Autodesk Inventor part; units mm, degrees
ref_plane "YZ Plane" through (0, 0, 0) normal (1, 0, 0) x (0, 1, 0)
ref_plane "XZ Plane" through (0, 0, 0) normal (0, 1, 0) x (-1, 0, 0)
ref_plane "XY Plane" through (0, 0, 0) normal (0, 0, 1) x (1, 0, 0)
sketch "スケッチ1" plane through (0, 0, 0) normal (0, 0, 1) x (1, 0, 0)
  circle A0 centre (0, 0) radius 3
  circle A1 centre (0, 40) radius 1.25
  circle A2 centre (0, 40) radius 3
  circle A3 centre (0, 0) radius 5
  line L0 (0, 5) -> (0, 37)
  line L1 (-2.9962, 40.15) -> (-4.9937, 0.25)
  dimension "d0" = 6
  dimension "d1" = 2.5
  dimension "d2" = 40
  dimension "d3" = 6
  dimension "d4" = 10
extrude "押し出し1" add sketch "スケッチ1" along normal blind 3
sketch "スケッチ2" plane through (0, 0, 3) normal (0, 0, 1) x (1, 0, 0)
  circle A0 centre (0, 0) radius 3
  circle A1 centre (0, 40) radius 1.25
  arc A2 (0, 37) -> (-2.9962, 40.15) centre (0, 40) ccw
  line L0 (-2.9962, 40.15) -> (-4.9937, 0.25)
  arc A3 (-4.9937, 0.25) -> (0, 5) centre (0, 0) ccw
  line L1 (0, 5) -> (0, 37)
  circle A4 centre (0, 0) radius 3
  circle A5 centre (-32.1289, 23.8272) radius 1.25
  line L2 (-4.0161, 2.9784) -> (-4.827, 3.5798)
  arc A6 (-30.4645, 26.3232) -> (-29.7192, 22.0402) centre (-32.1289, 23.8272) ccw
  line L3 (-4.5534, 9.0458) -> (2.7739, 4.16)
  arc A7 (-4.0161, 2.9784) -> (2.7739, 4.16) centre (0, 0) ccw
extrude "押し出し2" [suppressed]
sketch "スケッチ4" plane through (0, 0, 3) normal (0, 0, 1) x (1, 0, 0)
  line L0 (-4.9937, 0.25) -> (-2.9962, 40.15)
  arc A0 (0, 37) -> (-2.9962, 40.15) centre (0, 40) ccw
  line L1 (0, 37) -> (0, 5)
  circle A1 centre (0, 40) radius 1.25
  circle A2 centre (-27.9404, 11.376) radius 3
  circle A3 centre (0, 40) radius 1.25
  line L2 (-3.1661, 36.7564) -> (-2.0955, 37.8532)
  arc A4 (2.2489, 38.0144) -> (-2.0955, 37.8532) centre (0, 40) ccw
  line L3 (2.2489, 38.0144) -> (-3.4249, 31.5882)
  arc A5 (-24.4479, 14.954) -> (-24.1923, 8.0667) centre (-27.9404, 11.376) ccw
  circle A6 centre (0, 0) radius 3
  arc A7 (-4.9937, 0.25) -> (0, 5) centre (0, 0) ccw
extrude "押し出し3" [suppressed]
sketch "スケッチ5" plane through (0, 0, 3) normal (0, 0, 1) x (1, 0, 0)
  circle A0 centre (0, 0) radius 3
  circle A1 centre (0, 40) radius 1.25
  arc A2 (0, 37) -> (-2.9962, 40.15) centre (0, 40) ccw
  line L0 (-2.9962, 40.15) -> (-4.9937, 0.25)
  arc A3 (-4.9937, 0.25) -> (0, 5) centre (0, 0) ccw
  line L1 (0, 5) -> (0, 37)
  line L2 (0, 31) -> (3, 31)
  line L3 (3, 31) -> (3, 25)
  line L4 (3, 25) -> (0, 25)
  line L5 (0, 17) -> (3, 17)
  line L6 (3, 17) -> (3, 11)
  line L7 (3, 11) -> (0, 11)
  circle A4 centre (1.5, 14) radius 0.85
  circle A5 centre (1.5, 28) radius 0.85
  point P0 (1.5, 31)
  point P1 (1.5, 17)
  point P2 (3, 28)
  point P3 (3, 14)
  dimension "d12" = 6
  dimension "d13" = 3
  dimension "d14" = 8
  dimension "d15" = 6
  dimension "d16" = 6
  dimension "d19" = 1.7
extrude "押し出し4" add sketch "スケッチ5" against normal blind 3 contours L2 L3 L4 L1 | L5 L6 L7 L1
equation "\"d15\" = d16"
properties part number "link1"
Read the model definition and answer for the solid it produces. Units are mm, in the model's axes. A direction names the side the tool comes from. Coordinates: 2 decimals unless noted, no trailing zeros. Loops run counter-clockwise (first coordinate to the right, second up) from the corner with the lowest first, then second, coordinate; pieces in that order, holes last.
Q1. Consider probe 1 along X at (y, z) = (1.5, 0.55); probe 2 along Y at (x, z) = (0.5, 2.5); probe 3 along X at (y, z) = (39, 1.2). Determine where each line is inside the solid, lowest interval first.
Q2. Which of the six approach directions +Z, -Z, +X, -X, +Y, -Y give full straight-line access (tool end or side, diameter ignored) to faces 5 (the face through (3, 28, 2)), 6 (the face through (-1, 19, 0)), 7 (the face through (1, 31, 2))?
Q3. The part is cut by section A-A on x = -1.75. Write down the section's boundary in (y, z), and give its area (3 significant figures).
Q4. The part is cut by section D-D on y = 33. Write down the section's boundary in (x, z).
Q5. Each of these flat-tipped pins is pushed along its axis until it touches: pin 1 Ø1.5 at (x, z) = (1, 1) entering from -Y; pin 2 Ø0.9 at (y, z) = (26.5, 1.5) entering from +X; pin 3 Ø1.5 at (y, z) = (21.5, 1) entering from +X; pin 4 Ø1.5 at (x, y) = (1.5, 35.5) entering from -Z. Where does it stop, or does it pass through?
Q6. The part is cut by section B-B on y = 28. Write down the section's boundary in (x, z), and give its area (3 significant figures).
Q7. The mould has two halves that part along Y. Classify faces 1 (the face through (-3.98, 20.48, 1.48)), 2 (the face through (0.577, 41.109, 1.479)), 3 (the face through (0, 8, 1)), 4 (the face through (3, 14, 2)): +Y half, -Y half, draft (parallel to the pull), parting line (faces both ways), or undercut.
Q8. The part is cut by section C-C on z = 0.6. Write down the section's boundary in (x, y).
Results below:
1. probe 1: x = -4.93 to -2.6, 2.6 to 4.77
1. probe 2: y = -4.97 to -2.96, 2.96 to 4.97, 11 to 17, 25 to 31, 37.04 to 38.85, 41.15 to 42.96
1. probe 3: x = -3.05 to -0.75, 0.75 to 2.83
2. face 5: +Z, -Z, +X, +Y
2. face 6: -Z, +X, -X, +Y, -Y
2. face 7: +Z, -Z, +X
3. outline: (-4.68, 0) - (-2.44, 0) - (-2.44, 3) - (-4.68, 3) - close; (2.44, 0) - (42.44, 0) - (42.44, 3) - (2.44, 3) - close
3. area: 127 mm2
4. outline: (-3.35, 0) - (0, 0) - (0, 3) - (-3.35, 3) - close
5. pin 1: stops at y = -4.99
5. pin 2: stops at x = 3
5. pin 3: stops at x = 0
5. pin 4: passes through
6. outline: (-3.6, 0) - (0.65, 0) - (0.65, 3) - (-3.6, 3) - close; (2.35, 0) - (3, 0) - (3, 3) - (2.35, 3) - close
6. area: 14.7 mm2
7. face 1: +Y half
7. face 2: undercut
7. face 3: undercut
7. face 4: draft
8. outline: (-4.99, 0.25) arc R5 ccw (long way) to (0, 5) - (0, 11) - (3, 11) - (3, 17) - (0, 17) - (0, 25) - (3, 25) - (3, 31) - (0, 31) - (0, 37) arc R3 ccw (long way) to (-3, 40.15) - close; hole circle Ø6 at (0, 0); hole circle Ø2.5 at (0, 40); hole circle Ø1.7 at (1.5, 14); hole circle Ø1.7 at (1.5, 28)
